Could you check a few things on this model? Use its own coordinates, in mm. A direction names the side the tool comes from. Give positions to 0.01 mm unless a question says otherwise; leave off trailing zeros. Order: outer loops, then holes, each group sorted by start corner. A loop starts at its lowest first (then second) coordinate and runs counter-clockwise, first axis right, second up. Notation, with made-up numbers: M 12.5,67 L 54.5,67 A22 cw 54.5,99 Z; hole C 36,25 d4. An arc over 180 degrees is marked long. Return JSON: item names as keys, results as strings. Group by question number.
```python
from build123d import *

# Parameters (mm, degrees)
SKETCH4_W           = 413.09178157
SKETCH4_H           = 413.09178157
BOSS_EXTRUDE3_DEPTH = 6.604
SKETCH6_R           = 77.79258
CUT_EXTRUDE1_DEPTH  = 6.604
CUT_EXTRUDE2_DEPTH  = 6.604
CUT_EXTRUDE3_DEPTH  = 6.604


with BuildPart() as part:
    # Sketch4 → Boss-Extrude3 (new body)
    with BuildSketch(Plane(origin=(0, 0, 0), x_dir=(1, 0, 0), z_dir=(0, 1, 0))):
        Rectangle(SKETCH4_W, SKETCH4_H)
    extrude(amount=BOSS_EXTRUDE3_DEPTH)

    # Sketch6 → Cut-Extrude1 (cut)
    with BuildSketch(Plane(origin=(0, 6.604, 0), x_dir=(1, 0, 0), z_dir=(0, 1, 0))):
        Circle(SKETCH6_R)
    extrude(amount=-CUT_EXTRUDE1_DEPTH, mode=Mode.SUBTRACT)

    # Sketch8 → Cut-Extrude2 (cut)
    with BuildSketch(Plane(origin=(0, 6.604, 0), x_dir=(1, 0, 0), z_dir=(0, 1, 0))):
        Polygon((-111.193531291, -106.595640157), (106.595640157, 111.193531291), (111.193531291, 106.595640157), (-106.595640157, -111.193531291), align=None)
    extrude(amount=-CUT_EXTRUDE2_DEPTH, mode=Mode.SUBTRACT)

    # Sketch9 → Cut-Extrude3 (cut)
    with BuildSketch(Plane(origin=(0, 6.604, 0), x_dir=(1, 0, 0), z_dir=(0, 1, 0))):
        Polygon((111.202511547, -106.586659901), (-106.586659901, 111.202511547), (-111.202511547, 106.586659901), (106.586659901, -111.202511547), align=None)
    extrude(amount=-CUT_EXTRUDE3_DEPTH, mode=Mode.SUBTRACT)


solid = part.part
```
1. Imagine slicing it at A-A, the plane x = -63. Please give me the cut outline in (y, z).
2. Which directions (+Z, -Z, +X, -X, +Y, -Y) give clear straight access to the entire face, cutting with the end or side of a thin tool? Please do faces 3 (the cylindrical face through (77.79, 3.35, 0.8)), 4 (the flat face through (89, 0, -3)).
3. Imagine slicing it at D-D, the plane x = 10. Please give me the cut outline in (y, z).
4. I need wall thicknesses on L1, parallel to Z at x = 99.5, y = 0.75; L2, parallel to Z at x = 71, y = 0.5; L3, parallel to X at y = 5, z = 104. Which ranges of each line are inside material? Lowest first, please. Write a range as from..to.
5. Imagine slicing it at B-B, the plane y = 5. Please give me the cut outline in (x, z).
6. If we mould it in two halves opening along X, with no side actions, what happens to faces 1 (the flat face through (89, 6.604, -3)), 2 (the cylindrical face through (-0.82, 3.35, 77.79))? For each: pulls with the +X half, pulls with the -X half, needs draft (parallel to the pull), parting line crosses it, or undercut.
7. Imagine slicing it at C-C, the plane z = 17.5. Please give me the cut outline in (x, y), plus the area to 3 significant figures.
Values:
{
 "1": {"outline": "M 0,-206.55 L 6.6,-206.55 L 6.6,-67.62 L 0,-67.62 Z; M 0,-58.38 L 6.6,-58.38 L 6.6,-45.64 L 0,-45.64 Z; M 0,45.64 L 6.6,45.64 L 6.6,58.4 L 0,58.4 Z; M 0,67.6 L 6.6,67.6 L 6.6,206.55 L 0,206.55 Z"},
 "2": {"face 3": "+Y, -Y", "face 4": "+Z, -Z, +X, -X, -Y"},
 "3": {"outline": "M 0,-206.55 L 6.6,-206.55 L 6.6,-77.15 L 0,-77.15 Z; M 0,77.15 L 6.6,77.15 L 6.6,206.55 L 0,206.55 Z"},
 "4": {"L1": "z = -206.55..-104.1, -94.9..94.88, 104.12..206.55", "L2": "z = -206.55..-75.6, -66.4..-31.79, 31.79..66.38, 75.62..206.55", "L3": "x = -206.55..-108.6, -99.4..99.38, 108.62..206.55"},
 "5": {"outline": "M -206.55,-206.55 L 206.55,-206.55 L 206.55,206.55 L -206.55,206.55 Z; hole M -111.2,-106.59 L -106.59,-111.2 L -52.65,-57.27 A77.79 ccw 52.66,-57.26 L 106.6,-111.19 L 111.19,-106.6 L 57.26,-52.66 A77.79 ccw 57.27,52.65 L 111.2,106.59 L 106.59,111.2 L 52.65,57.27 A77.79 ccw -52.66,57.26 L -106.6,111.19 L -111.19,106.6 L -57.26,52.66 A77.79 ccw -57.27,-52.65 Z"},
 "6": {"face 1": "needs draft", "face 2": "undercut"},
 "7": {"outline": "M -206.55,0 L -75.8,0 L -75.8,6.6 L -206.55,6.6 Z; M 75.8,0 L 206.55,0 L 206.55,6.6 L 75.8,6.6 Z", "area": "1,730 mm²"}
}
